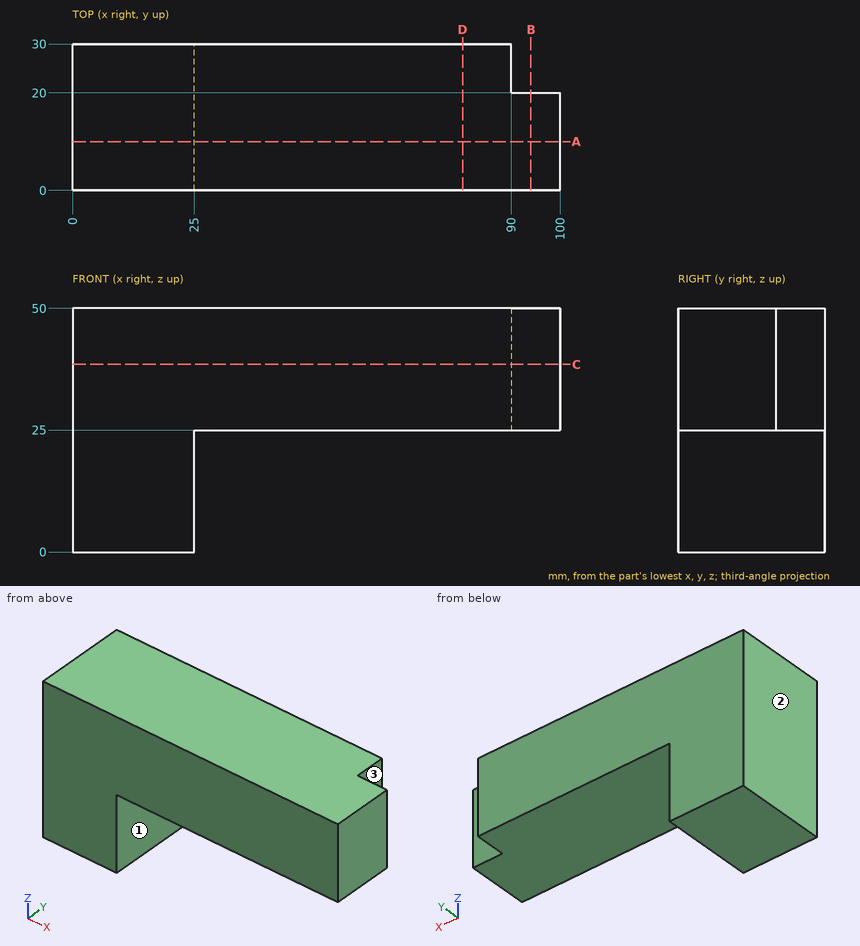
Design review of the part shown in the three views and the two pictorial views. Dimensions are in mm from the part's minimum x, y and z. A direction names the side the tool comes from. Round coordinates to 2 decimals unless told otherwise and drop trailing zeros. Write each loop counter-clockwise with the first axis right and the second up, starting at its lowest first coordinate (ties: lowest second). Pieces come first, ordered by that corner, then holes. Notation, with made-up numbers: (55, 20.5) -> (64, 20.5) arc R25 cw to (64, 50.5) -> close; hole circle Ø4 at (53, -28). An arc over 180 degrees is marked (long way). Write item = value, one per line. Start each with the question number.
1) Take a section at D-D, the plane x = 80. State the section outline as (y, z) points.
2) Take a section at A-A, the plane y = 10. State the section outline as (x, z) points, plus the area to 4 significant figures.
3) Take a section at C-C, the plane z = 38.5. State the section outline as (x, y) points.
4) Tool access review of the marked faces 1, 2 and 3: name each direction out of +Z, -Z, +X, -X, +Y, -Y from which nothing blocks a thin tool from reaching the whole face with its end or side.
5) Clearance check with flat-ended pins moving along their axes: pin 1 (8 mm diameter, centred on x = 96.5, z = 33.5, fed in from +Y); pin 2 (3 mm diameter, centred on y = 17, z = 6, fed in from +X); pin 3 (9 mm diameter, centred on x = 79.5, y = 19, fed in from -Z). State where each tip first meets the part, or that it passes through.
6) Wall thickness on probe 1 along Z at (x, y) = (92, 5.75); probe 2 along X at (y, z) = (17.25, 19.5); probe 3 along X at (y, z) = (27.25, 35): over which ranges is each line inside the solid? List them lowest first. Write a range as from..to.
7) Take a section at B-B, the plane x = 94. State the section outline as (y, z) points, plus the area to 3 significant figures.
Results list:
q1.outline = (0, 25) -> (30, 25) -> (30, 50) -> (0, 50) -> close
q2.outline = (0, 0) -> (25, 0) -> (25, 25) -> (100, 25) -> (100, 50) -> (0, 50) -> close
q2.area = 3,125 mm²
q3.outline = (0, 0) -> (100, 0) -> (100, 20) -> (90, 20) -> (90, 30) -> (0, 30) -> close
q4.face_1 = -Z, +X, +Y, -Y
q4.face_2 = +Z, -Z, -X, +Y, -Y
q4.face_3 = +Z, -Z, +X, +Y
q5.pin_1 = 20
q5.pin_2 = 25
q5.pin_3 = 25
q6.probe_1 = 25..50
q6.probe_2 = 0..25
q6.probe_3 = 0..90
q7.outline = (0, 25) -> (20, 25) -> (20, 50) -> (0, 50) -> close
q7.area = 500 mm²
